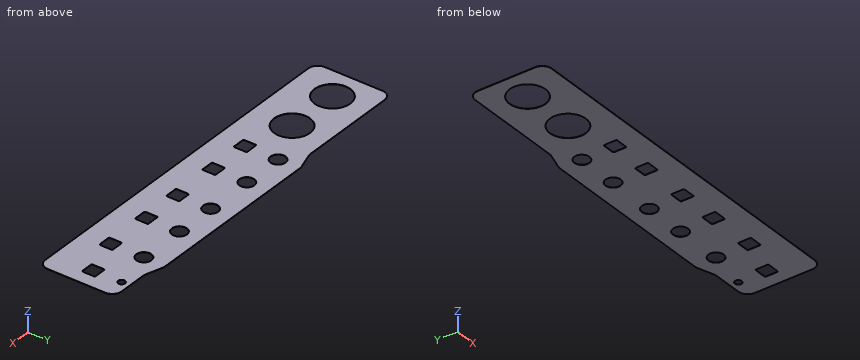
from build123d import *

# Parameters (mm, degrees)
PRINTED_FILM_START              = 14.65
PRINTED_FILM_DEPTH              = 0.15
OPENING_BNC_CHANNEL_0_START     = 14.9
OPENING_BNC_CHANNEL_0_PROFILE_R = 9.5
OPENING_BNC_CHANNEL_0_DEPTH     = 0.35
OPENING_BNC_CHANNEL_1_START     = 14.9
OPENING_BNC_CHANNEL_1_PROFILE_R = 9.5
OPENING_BNC_CHANNEL_1_DEPTH     = 0.35
OPENING_LED_RUN_START           = 14.9
OPENING_LED_RUN_PROFILE_R       = 1.8
OPENING_LED_RUN_DEPTH           = 0.35
OPENING_FUNC_START              = 14.9
OPENING_FUNC_PROFILE_R          = 4
OPENING_FUNC_DEPTH              = 0.35
OPENING_TRG_MODE_START          = 14.9
OPENING_TRG_MODE_DEPTH          = 0.35
OPENING_CURSOR_START            = 14.9
OPENING_CURSOR_DEPTH            = 0.35
OPENING_EN_CH1_START            = 14.9
OPENING_EN_CH1_DEPTH            = 0.35
OPENING_TRG_START               = 14.9
OPENING_TRG_PROFILE_R           = 4
OPENING_TRG_DEPTH               = 0.35
OPENING_TIME_START              = 14.9
OPENING_TIME_PROFILE_R          = 4
OPENING_TIME_DEPTH              = 0.35
OPENING_SET_CH1_START           = 14.9
OPENING_SET_CH1_PROFILE_R       = 4
OPENING_SET_CH1_DEPTH           = 0.35
OPENING_SET_CH0_START           = 14.9
OPENING_SET_CH0_PROFILE_R       = 4
OPENING_SET_CH0_DEPTH           = 0.35
OPENING_RUN_STOP_START          = 14.9
OPENING_RUN_STOP_DEPTH          = 0.35
OPENING_MENU_BACK_START         = 14.9
OPENING_MENU_BACK_DEPTH         = 0.35
OPENING_EN_CH0_START            = 14.9
OPENING_EN_CH0_DEPTH            = 0.35


with BuildPart() as part:
    # Printed_film_profile → Printed_film (new body)
    with BuildSketch(Plane.XY.offset(PRINTED_FILM_START)):
        with BuildLine():
            Line((2.4, -6.6), (187.6, -6.6))
            ThreePointArc((187.6, -6.6), (191.135533906, -5.135533906), (192.6, -1.6))
            Line((192.6, -1.6), (192.6, 28.8))
            ThreePointArc((192.6, 28.8), (191.135533906, 32.335533906), (187.6, 33.8))
            Line((187.6, 33.8), (172.557224923, 33.8))
            ThreePointArc((172.557224923, 33.8), (171.808537122, 33.856371113), (171.076731067, 34.024213369))
            Line((171.076731067, 34.024213369), (162.523268933, 36.675786631))
            ThreePointArc((162.523268933, 36.675786631), (161.791462878, 36.843628887), (161.042775077, 36.9))
            Line((161.042775077, 36.9), (66.157224923, 36.9))
            ThreePointArc((66.157224923, 36.9), (65.408537122, 36.843628887), (64.676731067, 36.675786631))
            Line((64.676731067, 36.675786631), (56.123268933, 34.024213369))
            ThreePointArc((56.123268933, 34.024213369), (55.391462878, 33.856371113), (54.642775077, 33.8))
            Line((54.642775077, 33.8), (2.4, 33.8))
            ThreePointArc((2.4, 33.8), (-1.135533906, 32.335533906), (-2.6, 28.8))
            Line((-2.6, 28.8), (-2.6, -1.6))
            ThreePointArc((-2.6, -1.6), (-1.135533906, -5.135533906), (2.4, -6.6))
        make_face()
    extrude(amount=PRINTED_FILM_DEPTH)

    # Opening_BNC_Channel_0_profile → Opening_BNC_Channel_0 (cut)
    with BuildSketch(Plane.XY.offset(OPENING_BNC_CHANNEL_0_START)):
        with Locations((13.5, 14.5)):
            Circle(OPENING_BNC_CHANNEL_0_PROFILE_R)
    extrude(amount=-OPENING_BNC_CHANNEL_0_DEPTH, mode=Mode.SUBTRACT)

    # Opening_BNC_Channel_1_profile → Opening_BNC_Channel_1 (cut)
    with BuildSketch(Plane.XY.offset(OPENING_BNC_CHANNEL_1_START)):
        with Locations((41.9, 14.5)):
            Circle(OPENING_BNC_CHANNEL_1_PROFILE_R)
    extrude(amount=-OPENING_BNC_CHANNEL_1_DEPTH, mode=Mode.SUBTRACT)

    # Opening_LED_RUN_profile → Opening_LED_RUN (cut)
    with BuildSketch(Plane.XY.offset(OPENING_LED_RUN_START)):
        with Locations((181.9, 29.5)):
            Circle(OPENING_LED_RUN_PROFILE_R)
    extrude(amount=-OPENING_LED_RUN_DEPTH, mode=Mode.SUBTRACT)

    # Opening_FUNC_profile → Opening_FUNC (cut)
    with BuildSketch(Plane.XY.offset(OPENING_FUNC_START)):
        with Locations((160.9, 25.5)):
            Circle(OPENING_FUNC_PROFILE_R)
    extrude(amount=-OPENING_FUNC_DEPTH, mode=Mode.SUBTRACT)

    # Opening_TRG_MODE_profile → Opening_TRG_MODE (cut)
    with BuildSketch(Plane.XY.offset(OPENING_TRG_MODE_START)):
        with BuildLine():
            Line((133, 4.5), (138.8, 4.5))
            ThreePointArc((138.8, 4.5), (139.224264069, 4.675735931), (139.4, 5.1))
            Line((139.4, 5.1), (139.4, 10.9))
            ThreePointArc((139.4, 10.9), (139.224264069, 11.324264069), (138.8, 11.5))
            Line((138.8, 11.5), (133, 11.5))
            ThreePointArc((133, 11.5), (132.575735931, 11.324264069), (132.4, 10.9))
            Line((132.4, 10.9), (132.4, 5.1))
            ThreePointArc((132.4, 5.1), (132.575735931, 4.675735931), (133, 4.5))
        make_face()
    extrude(amount=-OPENING_TRG_MODE_DEPTH, mode=Mode.SUBTRACT)

    # Opening_CURSOR_profile → Opening_CURSOR (cut)
    with BuildSketch(Plane.XY.offset(OPENING_CURSOR_START)):
        with BuildLine():
            Line((111, 4.5), (116.8, 4.5))
            ThreePointArc((116.8, 4.5), (117.224264069, 4.675735931), (117.4, 5.1))
            Line((117.4, 5.1), (117.4, 10.9))
            ThreePointArc((117.4, 10.9), (117.224264069, 11.324264069), (116.8, 11.5))
            Line((116.8, 11.5), (111, 11.5))
            ThreePointArc((111, 11.5), (110.575735931, 11.324264069), (110.4, 10.9))
            Line((110.4, 10.9), (110.4, 5.1))
            ThreePointArc((110.4, 5.1), (110.575735931, 4.675735931), (111, 4.5))
        make_face()
    extrude(amount=-OPENING_CURSOR_DEPTH, mode=Mode.SUBTRACT)

    # Opening_EN_CH1_profile → Opening_EN_CH1 (cut)
    with BuildSketch(Plane.XY.offset(OPENING_EN_CH1_START)):
        with BuildLine():
            Line((85.6, 4.5), (91.4, 4.5))
            ThreePointArc((91.4, 4.5), (91.824264069, 4.675735931), (92, 5.1))
            Line((92, 5.1), (92, 10.9))
            ThreePointArc((92, 10.9), (91.824264069, 11.324264069), (91.4, 11.5))
            Line((91.4, 11.5), (85.6, 11.5))
            ThreePointArc((85.6, 11.5), (85.175735931, 11.324264069), (85, 10.9))
            Line((85, 10.9), (85, 5.1))
            ThreePointArc((85, 5.1), (85.175735931, 4.675735931), (85.6, 4.5))
        make_face()
    extrude(amount=-OPENING_EN_CH1_DEPTH, mode=Mode.SUBTRACT)

    # Opening_TRG_profile → Opening_TRG (cut)
    with BuildSketch(Plane.XY.offset(OPENING_TRG_START)):
        with Locations((135.9, 25.5)):
            Circle(OPENING_TRG_PROFILE_R)
    extrude(amount=-OPENING_TRG_DEPTH, mode=Mode.SUBTRACT)

    # Opening_TIME_profile → Opening_TIME (cut)
    with BuildSketch(Plane.XY.offset(OPENING_TIME_START)):
        with Locations((113.9, 25.5)):
            Circle(OPENING_TIME_PROFILE_R)
    extrude(amount=-OPENING_TIME_DEPTH, mode=Mode.SUBTRACT)

    # Opening_SET_CH1_profile → Opening_SET_CH1 (cut)
    with BuildSketch(Plane.XY.offset(OPENING_SET_CH1_START)):
        with Locations((88.4, 25.5)):
            Circle(OPENING_SET_CH1_PROFILE_R)
    extrude(amount=-OPENING_SET_CH1_DEPTH, mode=Mode.SUBTRACT)

    # Opening_SET_CH0_profile → Opening_SET_CH0 (cut)
    with BuildSketch(Plane.XY.offset(OPENING_SET_CH0_START)):
        with Locations((66.4, 25.5)):
            Circle(OPENING_SET_CH0_PROFILE_R)
    extrude(amount=-OPENING_SET_CH0_DEPTH, mode=Mode.SUBTRACT)

    # Opening_RUN_STOP_profile → Opening_RUN_STOP (cut)
    with BuildSketch(Plane.XY.offset(OPENING_RUN_STOP_START)):
        with BuildLine():
            Line((179, 11), (184.8, 11))
            ThreePointArc((184.8, 11), (185.224264069, 11.175735931), (185.4, 11.6))
            Line((185.4, 11.6), (185.4, 17.4))
            ThreePointArc((185.4, 17.4), (185.224264069, 17.824264069), (184.8, 18))
            Line((184.8, 18), (179, 18))
            ThreePointArc((179, 18), (178.575735931, 17.824264069), (178.4, 17.4))
            Line((178.4, 17.4), (178.4, 11.6))
            ThreePointArc((178.4, 11.6), (178.575735931, 11.175735931), (179, 11))
        make_face()
    extrude(amount=-OPENING_RUN_STOP_DEPTH, mode=Mode.SUBTRACT)

    # Opening_MENU_BACK_profile → Opening_MENU_BACK (cut)
    with BuildSketch(Plane.XY.offset(OPENING_MENU_BACK_START)):
        with BuildLine():
            Line((158.1, 4.5), (163.9, 4.5))
            ThreePointArc((163.9, 4.5), (164.324264069, 4.675735931), (164.5, 5.1))
            Line((164.5, 5.1), (164.5, 10.9))
            ThreePointArc((164.5, 10.9), (164.324264069, 11.324264069), (163.9, 11.5))
            Line((163.9, 11.5), (158.1, 11.5))
            ThreePointArc((158.1, 11.5), (157.675735931, 11.324264069), (157.5, 10.9))
            Line((157.5, 10.9), (157.5, 5.1))
            ThreePointArc((157.5, 5.1), (157.675735931, 4.675735931), (158.1, 4.5))
        make_face()
    extrude(amount=-OPENING_MENU_BACK_DEPTH, mode=Mode.SUBTRACT)

    # Opening_EN_CH0_profile → Opening_EN_CH0 (cut)
    with BuildSketch(Plane.XY.offset(OPENING_EN_CH0_START)):
        with BuildLine():
            Line((63.5, 4.5), (69.3, 4.5))
            ThreePointArc((69.3, 4.5), (69.724264069, 4.675735931), (69.9, 5.1))
            Line((69.9, 5.1), (69.9, 10.9))
            ThreePointArc((69.9, 10.9), (69.724264069, 11.324264069), (69.3, 11.5))
            Line((69.3, 11.5), (63.5, 11.5))
            ThreePointArc((63.5, 11.5), (63.075735931, 11.324264069), (62.9, 10.9))
            Line((62.9, 10.9), (62.9, 5.1))
            ThreePointArc((62.9, 5.1), (63.075735931, 4.675735931), (63.5, 4.5))
        make_face()
    extrude(amount=-OPENING_EN_CH0_DEPTH, mode=Mode.SUBTRACT)


solid = part.part
The model under review builds one solid part; all positions refer to its coordinate system, in mm. Coordinates: 2 decimals unless noted, no trailing zeros. Loops run counter-clockwise (first coordinate to the right, second up) from the corner with the lowest first, then second, coordinate; pieces in that order, holes last. Notation, with made-up numbers: M -21,-16 L 22,-16 A13 ccw 22,2 Z; hole C -17,48 d6. An arc over 180 degrees is marked long. Put each result on its own line as item: value. Start each with the question number.
Q1. Wall thickness on line 1 (Y direction, x = 88.4, z = 14.7); line 2 (Y direction, x = 41.9, z = 14.7); line 3 (X direction, y = 27, z = 14.7): over which ranges is each line inside the solid? List them lowest first.
Q2. Add section C-C (y = 7.5). Count the separate pieces of the cut face and the enclosed holes in it, and give its area (3 significant figures).
Q3. Clearance check with a flat-ended pin moving along its axis: pin 1 (5 mm diameter, centred on x = 66.4, y = 25.5, fed in from +Z). State where the tip first meets the part, or that it passes through.
Q4. Add section B-B (x = 181.9). Write out the cut boundary in (y, z).
Q5. Add section D-D (x = 88.4). Write out the cut boundary in (y, z).
Q6. Add section A-A (x = 41.9). Write out the cut boundary in (y, z).
Answers:
1. line 1: y = -6.6 to 4.5, 11.5 to 21.5, 29.5 to 36.9
1. line 2: y = -6.6 to 5, 24 to 33.8
1. line 3: x = -2.6 to 62.69, 70.11 to 84.69, 92.11 to 110.19, 117.61 to 132.19, 139.61 to 157.19, 164.61 to 192.6
2. separate pieces: 8
2. enclosed holes: 0
2. area: 20.2 mm^2
3. pin 1: passes through
4. outline: M -6.6,14.65 L 11,14.65 L 11,14.8 L -6.6,14.8 Z; M 18,14.65 L 27.7,14.65 L 27.7,14.8 L 18,14.8 Z; M 31.3,14.65 L 33.8,14.65 L 33.8,14.8 L 31.3,14.8 Z
5. outline: M -6.6,14.65 L 4.5,14.65 L 4.5,14.8 L -6.6,14.8 Z; M 11.5,14.65 L 21.5,14.65 L 21.5,14.8 L 11.5,14.8 Z; M 29.5,14.65 L 36.9,14.65 L 36.9,14.8 L 29.5,14.8 Z
6. outline: M -6.6,14.65 L 5,14.65 L 5,14.8 L -6.6,14.8 Z; M 24,14.65 L 33.8,14.65 L 33.8,14.8 L 24,14.8 Z
